Autodesk Inventor part; units mm, degrees
ref_plane "BODY5_XY" through (0, 0, 0) normal (0, 0, 1) x (1, 0, 0)
ref_plane "BODY5_YZ" through (0, 0, 0) normal (1, 0, 0) x (0, 1, 0)
ref_plane "BODY5_ZX" through (0, 0, 0) normal (0, 1, 0) x (0, 0, 1)
sketch "__1" plane through (0, 0, 0) normal (0, 0, 1) x (1, 0, 0)
  line L0 (-75.035, 43.97) -> (-75.035, 2)
  arc A0 (-75.035, 2) -> (-73.035, 0) centre (-73.035, 2) ccw
  line L1 (-73.035, 0) -> (73.035, 0)
  arc A1 (73.035, 0) -> (75.035, 2) centre (73.035, 2) ccw
  line L2 (75.035, 2) -> (75.035, 33.5658)
  arc A2 (75.035, 33.5658) -> (74.7421, 34.2729) centre (74.035, 33.5658) ccw
  line L3 (74.7421, 34.2729) -> (73.8708, 35.1442)
  arc A3 (73.285, 36.5584) -> (73.8708, 35.1442) centre (75.285, 36.5584) ccw
  line L4 (73.285, 36.5584) -> (73.285, 38.4016)
  arc A4 (73.8708, 39.8158) -> (73.285, 38.4016) centre (75.285, 38.4016) ccw
  line L5 (73.8708, 39.8158) -> (74.7421, 40.6871)
  arc A5 (74.7421, 40.6871) -> (75.035, 41.3942) centre (74.035, 41.3942) ccw
  line L6 (75.035, 41.3942) -> (75.035, 43.97)
  arc A6 (75.035, 43.97) -> (74.035, 44.97) centre (74.035, 43.97) ccw
  line L7 (74.035, 44.97) -> (70.2376, 44.97)
  arc A7 (68.1163, 45.8487) -> (70.2376, 44.97) centre (70.2376, 47.97) ccw
  line L8 (68.1163, 45.8487) -> (62.3737, 51.5913)
  arc A8 (62.3737, 51.5913) -> (60.2524, 52.47) centre (60.2524, 49.47) ccw
  line L9 (60.2524, 52.47) -> (37.485, 52.47)
  arc A9 (35.485, 54.47) -> (37.485, 52.47) centre (37.485, 54.47) ccw
  line L10 (35.485, 54.47) -> (35.485, 56.24)
  arc A10 (35.485, 56.24) -> (34.065, 57.96) centre (33.4947, 56.043) ccw
  line L11 (34.065, 57.96) -> (30.735, 58.57)
  line L12 (30.735, 58.57) -> (30.735, 61)
  arc A11 (30.735, 61) -> (29.735, 62) centre (29.735, 61) ccw
  line L13 (29.735, 62) -> (-29.735, 62)
  arc A12 (-29.735, 62) -> (-30.735, 61) centre (-29.735, 61) ccw
  line L14 (-30.735, 61) -> (-30.735, 58.57)
  line L15 (-30.735, 58.57) -> (-34.065, 57.96)
  arc A13 (-34.065, 57.96) -> (-35.485, 56.24) centre (-33.4947, 56.043) ccw
  line L16 (-35.485, 56.24) -> (-35.485, 54.47)
  arc A14 (-37.485, 52.47) -> (-35.485, 54.47) centre (-37.485, 54.47) ccw
  line L17 (-37.485, 52.47) -> (-60.2524, 52.47)
  arc A15 (-60.2524, 52.47) -> (-62.3737, 51.5913) centre (-60.2524, 49.47) ccw
  line L18 (-62.3737, 51.5913) -> (-68.1163, 45.8487)
  arc A16 (-70.2376, 44.97) -> (-68.1163, 45.8487) centre (-70.2376, 47.97) ccw
  line L19 (-70.2376, 44.97) -> (-74.035, 44.97)
  arc A17 (-74.035, 44.97) -> (-75.035, 43.97) centre (-74.035, 43.97) ccw
  circle A18 centre (0, 31.48) radius 16.5
extrude "Extrusion1" add sketch "__1" along normal blind 15
sketch "__3" plane through (0, 0, 0) normal (0, 1, 0) x (-1, 0, 0)
  line L0 (80, 6.03) -> (80, 18)
  line L1 (80, 18) -> (-80, 18)
  line L2 (-80, 18) -> (-80, 6.03)
  line L3 (-80, 6.03) -> (-30.735, 7.55)
  line L4 (-30.735, 7.55) -> (-30.28, 15)
  line L5 (-30.28, 15) -> (30.28, 15)
  line L6 (30.28, 15) -> (30.735, 7.55)
  line L7 (30.735, 7.55) -> (80, 6.03)
extrude "Extrusion2" cut sketch "__3" along normal blind 61.97
sketch "__4" plane through (0, 0, 0) normal (1, 0, 0) x (0, 1, 0)
  line L0 (63.944, 20) -> (0, 20)
  line L1 (0, 20) -> (0, 0)
  line L2 (0, 0) -> (0.46, 15)
  line L3 (0.46, 15) -> (61.51, 15)
  line L4 (61.51, 15) -> (61.97, 0)
  line L5 (61.97, 0) -> (63.944, 0)
  line L6 (63.944, 0) -> (63.944, 20)
extrude "Extrusion3" cut sketch "__4" along normal mid plane 150.07
ref_plane "BODY5_XY" through (0, 0, 0) normal (0, 0, 1) x (1, 0, 0)
ref_plane "BODY5_YZ" through (0, 0, 0) normal (1, 0, 0) x (0, 1, 0)
ref_plane "BODY5_ZX" through (0, 0, 0) normal (0, 1, 0) x (0, 0, 1)
ref_plane "MD1_XY" through (0, 31.48, 15) normal (0, 0, -1) x (1, 0, 0)
ref_plane "MD1_YZ" through (0, 31.48, 15) normal (1, 0, 0) x (0, -1, 0)
ref_plane "MD1_ZX" through (0, 31.48, 15) normal (0, -1, 0) x (0, 0, -1)
properties part number "ETH2-17-BC-L_5"
Build history of the part. All positions in model axes, mm. A direction names the side the tool comes from. Give positions to 0.01 mm unless a question says otherwise; leave off trailing zeros. Loops run counter-clockwise (first coordinate to the right, second up) from the corner with the lowest first, then second, coordinate; pieces in that order, holes last. Notation, with made-up numbers: (-26, -16) -> (29, -16) arc R33 cw to (29, 19) -> close; hole circle Ø9 at (-12, 83). An arc over 180 degrees is marked (long way). One line per question, with ' | ' between items. Start each with the question number.
1) Cut at A-A (y = 31.48). Give the cut face in (x, z) (3 decimals).
2) Probe L1, parallel to Y at x = 0, z = 6; L2, parallel to X at y = 29.5, z = 5.5 (3 decimals); L3, parallel to Z at x = 63, y = 9. List the from-to ranges inside material, lowest first.
3) 3-axis set-ups, long thin cutter, end or side, ignore diameter. For faces 1 (the flat face through (72, 44.97, 3)), 2 (the flat face through (-72, 44.97, 3)), 3 (the flat face through (30.51, 30.5, 11.22)): which of +Z, -Z, +X, -X, +Y, -Y reach the whole face in a straight line?
4) Cut at B-B (x = 0). Give the cut face in (y, z), plus the area to 3 significant figures.
5) Cut at D-D (z = 13). Give the cut face in (x, y).
6) Cut at C-C (y = 11). Give the cut face in (x, z) (3 decimals), plus the area to 3 significant figures.
7) Pin check, flat tips, straight feed: pin 1 (8 mm diameter, centred on x = -51.5, z = 3.5, fed in from +Y); pin 2 (2 mm diameter, centred on y = 49, z = 12, fed in from +X); pin 3 (1 mm diameter, centred on y = 39, z = 12, fed in from -X). Stop position of each tip, or through.
8) Two-plate mould, pull along X, no slides. Class faces 4 (the flat face through (-49, 52.47, 4)), 5 (the flat face through (75.035, 43, 3)), 6 (the cylindrical face through (-3.577, 47.588, 7.395)): released by +X, released by -X, zero draft, split by the parting line, or undercut.
Return value:
1) outline: (-75.035, 0) -> (-16.5, 0) -> (-16.5, 15) -> (-30.28, 15) -> (-30.735, 7.55) -> (-75.035, 6.183) -> close; (16.5, 0) -> (75.035, 0) -> (75.035, 6.183) -> (30.735, 7.55) -> (30.28, 15) -> (16.5, 15) -> close
2) L1: 0.18 to 14.98, 47.98 to 61.79 | L2: -75.035 to -16.381, 16.381 to 75.035 | L3: 0 to 6.55
3) face 1: +Z, -Z, +X, +Y | face 2: +Z, -Z, -X, +Y | face 3: +Z, +X, +Y, -Y
4) outline: (0, 0) -> (14.98, 0) -> (14.98, 15) -> (0.46, 15) -> close; (47.98, 0) -> (61.97, 0) -> (61.51, 15) -> (47.98, 15) -> close | area: 428 mm^2
5) outline: (-30.4, 0.4) -> (30.4, 0.4) -> (30.4, 61.57) -> (-30.4, 61.57) -> close; hole circle Ø33 at (0, 31.48)
6) outline: (-75.035, 0) -> (75.035, 0) -> (75.035, 6.183) -> (30.735, 7.55) -> (30.28, 15) -> (-30.28, 15) -> (-30.735, 7.55) -> (-75.035, 6.183) -> close | area: 1,530 mm^2
7) pin 1: y = 52.47 | pin 2: x = 30.52 | pin 3: x = -30.49
8) face 4: zero draft | face 5: released by +X | face 6: undercut
